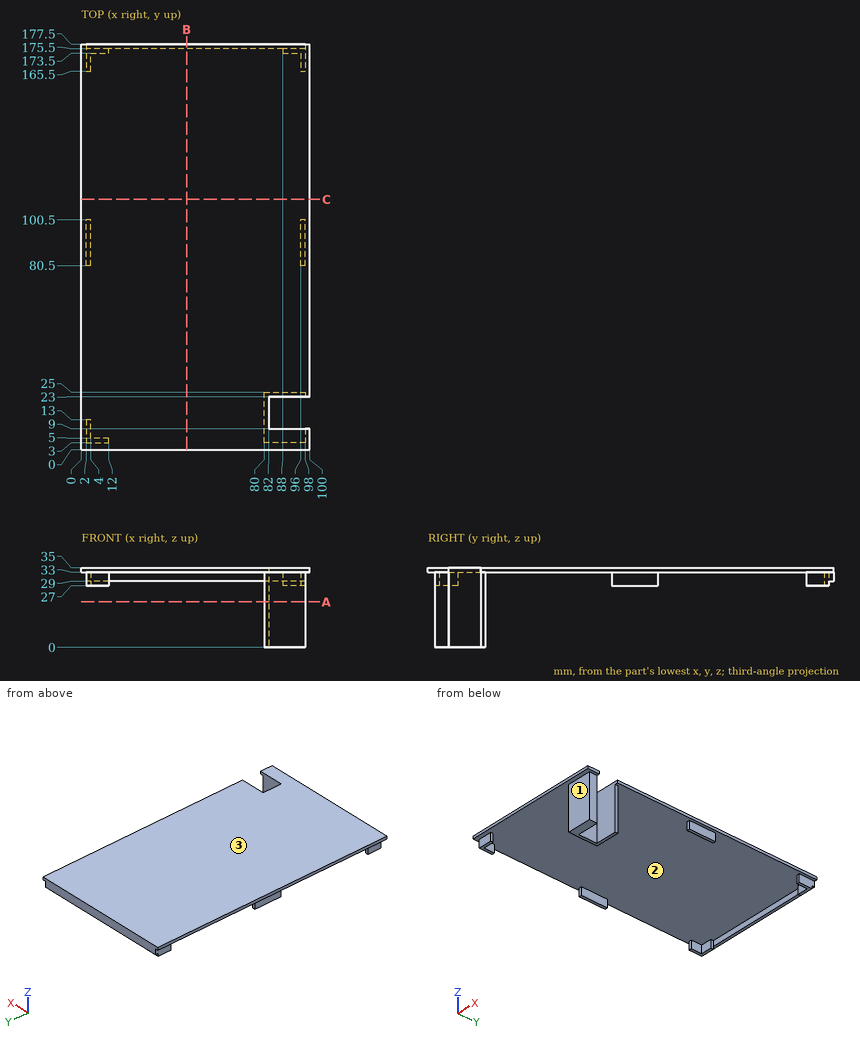
Design review of the part shown in the three views and the two pictorial views. Dimensions are in mm from the part's minimum x, y and z. Round coordinates to 2 decimals unless told otherwise and drop trailing zeros. Write each loop counter-clockwise with the first axis right and the second up, starting at its lowest first coordinate (ties: lowest second). Pieces come first, ordered by that corner, then holes.
1) Mouldability with a two-part tool opening along Y and no side actions: class the marked faces 1, 2 and 3 as +Y half, -Y half, draft (parallel to the pull), parting line (faces both ways), or undercut.
Answer below:
face 1: -Y half
face 2: undercut
face 3: draft
2) Take a section at A-A on z = 20. Give the boundary of the cut face in (x, y), then the cut area to 3 significant figures.
Answer below:
outline: (80, 3) - (98, 3) - (98, 9) - (82, 9) - (82, 23) - (98, 23) - (98, 25) - (80, 25) - close
area: 172 mm2
3) Insertion check: pin 1 Ø3 at (y, z) = (170.5, 30.5) entering from -X; pin 2 Ø3 at (y, z) = (7, 22.5) entering from +X; pin 3 Ø1 at (x, z) = (97, 30.5) entering from -Y; pin 4 Ø6 at (y, z) = (30, 8) entering from +X (3 decimals). Each pin has a flat end and moves straight along its axis. Give the tip position at first contact, or say it passes through.
Answer below:
pin 1: stops at x = 2
pin 2: stops at x = 98
pin 3: stops at y = 3
pin 4: passes through
4) Take a section at C-C on y = 109.5. Give the boundary of the cut face in (x, z).
Answer below:
outline: (0, 33) - (100, 33) - (100, 35) - (0, 35) - close
5) Take a section at B-B on x = 46. Give the boundary of the cut face in (y, z), then the cut area to 3 significant figures.
Answer below:
outline: (0, 33) - (175.5, 33) - (175.5, 29) - (177.5, 29) - (177.5, 35) - (0, 35) - close
area: 363 mm2
6) For line 1 along Y through (x, z) = (93, 25.5); line 2 along Z through (x, y) = (79.5, 15.5); line 3 along X through (y, z) = (20.5, 26), list the stretches that pass through material, from the lowest coordinate up.
Answer below:
line 1: y = 3 to 9, 23 to 25
line 2: z = 33 to 35
line 3: x = 80 to 82
